```python
from build123d import *

# Parameters (mm, degrees)
BOSS_EXTRUDE1_DEPTH = 11.176
SKETCH2_R           = 2.032
CUT_EXTRUDE1_DEPTH  = 26.73462306
SKETCH4_W           = 2.54
SKETCH4_H           = 6.858
CUT_EXTRUDE2_DEPTH  = 0.508
SKETCH5_W           = 2.54
SKETCH5_H           = 6.858
CUT_EXTRUDE3_DEPTH  = 0.508


with BuildPart() as part:
    # Sketch1 → Boss-Extrude1 (new body)
    with BuildSketch(Plane.XY):
        with BuildLine():
            Line((8.39837008, 0), (21.09837008, 0))
            Line((21.09837008, 0), (21.09837008, 6.35))
            Line((21.09837008, 6.35), (21.60637008, 6.35))
            Line((21.60637008, 6.35), (21.60637008, -0.508))
            Line((21.60637008, -0.508), (7.874, -0.508))
            ThreePointArc((7.874, -0.508), (0, 7.89037008), (-7.874, -0.508))
            Line((-7.874, -0.508), (-21.60637008, -0.508))
            Line((-21.60637008, -0.508), (-21.60637008, 6.35))
            Line((-21.60637008, 6.35), (-21.09837008, 6.35))
            Line((-21.09837008, 6.35), (-21.09837008, 0))
            Line((-21.09837008, 0), (-8.39837008, 0))
            ThreePointArc((-8.39837008, 0), (0, 8.39837008), (8.39837008, 0))
        make_face()
    extrude(amount=BOSS_EXTRUDE1_DEPTH)

    # Sketch2 → Cut-Extrude1 (cut, through all)
    with BuildSketch(Plane(origin=(0, 0, 0), x_dir=(1, 0, 0), z_dir=(0, 1, 0))):
        with Locations(Location((15.00237008, -5.588, 0), (0, 0, 270))):
            Circle(SKETCH2_R)
        with Locations(Location((-15.00237008, -5.588, 0), (0, 0, 90))):
            Circle(SKETCH2_R)
    extrude(amount=-CUT_EXTRUDE1_DEPTH, mode=Mode.SUBTRACT)

    # Sketch4 → Cut-Extrude2 (cut)
    with BuildSketch(Plane(origin=(21.60637008, 0, 0), x_dir=(0, 0, -1), z_dir=(1, 0, 0))):
        with Locations((-5.207, 2.921)):
            Rectangle(SKETCH4_W, SKETCH4_H)
    extrude(amount=-CUT_EXTRUDE2_DEPTH, mode=Mode.SUBTRACT)

    # Sketch5 → Cut-Extrude3 (cut)
    with BuildSketch(Plane.ZY.offset(21.60637008)):
        with Locations((5.969, 2.921)):
            Rectangle(SKETCH5_W, SKETCH5_H)
    extrude(amount=-CUT_EXTRUDE3_DEPTH, mode=Mode.SUBTRACT)


solid = part.part
```
Geometry check sheet. Reference: the model listing, model coordinates, mm. A direction names the side the tool comes from. Give positions to 0.01 mm unless a question says otherwise; leave off trailing zeros. Loops run counter-clockwise (first coordinate to the right, second up) from the corner with the lowest first, then second, coordinate; pieces in that order, holes last. Notation, with made-up numbers: M 0.5,-28 L 10.5,-28 A17 cw 10.5,-7 Z; hole C 9.25,66 d3. An arc over 180 degrees is marked long. Write item = value, one per line. Start each with the question number.
1. Tool access check on faces 1 (the face through (-21.606, 3, 9)), 2 (the face through (-13, 0, 4)). Record the directions out of +Z, -Z, +X, -X, +Y, -Y that give a thin tool (end or side, any length) a straight path to the whole face; none if there is none.
2. Section check A-A, the plane z = 5.5. Enter the section's corners in (x, y).
3. Draft check along X on faces 3 (the face through (21.606, 3, 2)), 4 (the face through (-1, 8, 0)), 5 (the face through (-21.606, 3, 2)), 6 (the face through (21.098, 3, 2)). Enter one of: +X half, -X half, draft (parallel to the pull), parting line (faces both ways), or undercut.
4. Section check C-C, the plane z = 9.75. Enter the section's corners in (x, y), plus the area to 3 significant figures.
5. Thickness scan on probe 1 along X at (y, z) = (4.5, 3); probe 2 along X at (y, z) = (4.75, 2.5); probe 3 along Y at (x, z) = (18, 5.25). Record the ranges inside material, lowest first.
6. Section check B-B, the plane y = 5.25. Enter the section's corners in (x, z), plus the area to 3 significant figures.
7. Section check D-D, the plane y = 1.25. Enter the section's corners in (x, z), plus the area to 3 significant figures.
8. Go/stop test with flat-tipped pins: P1, Ø5.5, axis at x = -15.5, z = 7.5, coming from the +Y side; P2, Ø5, axis at y = 2, z = 4, coming from the +X side; P3, Ø1, axis at x = -1, z = 5.5, coming from the +Y side; P4, Ø1.5, axis at x = -3.5, z = 1.5, coming from the -Y side. Record where each tip stops, or that it passes through.
Values follow:
q1.face_1 = +Z, -Z, -X, +Y, -Y
q1.face_2 = +Z, -Z, +Y
q2.outline = M -21.1,-0.51 L -17.03,-0.51 L -17.03,0 L -21.1,0 Z; M -12.97,-0.51 L -7.87,-0.51 A7.89 cw long 7.87,-0.51 L 12.97,-0.51 L 12.97,0 L 8.4,0 A8.4 ccw -8.4,0 L -12.97,0 Z; M 17.03,-0.51 L 21.1,-0.51 L 21.1,0 L 17.03,0 Z
q3.face_3 = +X half
q3.face_4 = draft
q3.face_5 = -X half
q3.face_6 = undercut
q4.outline = M -21.61,-0.51 L -7.87,-0.51 A7.89 cw long 7.87,-0.51 L 21.61,-0.51 L 21.61,6.35 L 21.1,6.35 L 21.1,0 L 8.4,0 A8.4 ccw -8.4,0 L -21.1,0 L -21.1,6.35 L -21.61,6.35 Z
q4.area = 33.4 mm^2
q5.probe_1 = -21.61 to -21.1, -7.09 to -6.48, 6.48 to 7.09, 21.1 to 21.61
q5.probe_2 = -21.61 to -21.1, -6.93 to -6.3, 6.3 to 6.93, 21.1 to 21.61
q5.probe_3 = -0.51 to 0
q6.outline = M -21.61,0 L -21.1,0 L -21.1,4.7 L -21.61,4.7 Z; M -21.61,7.24 L -21.1,7.24 L -21.1,11.18 L -21.61,11.18 Z; M -6.56,0 L -5.89,0 L -5.89,11.18 L -6.56,11.18 Z; M 5.89,0 L 6.56,0 L 6.56,11.18 L 5.89,11.18 Z; M 21.1,0 L 21.61,0 L 21.61,3.94 L 21.1,3.94 Z; M 21.1,6.48 L 21.61,6.48 L 21.61,11.18 L 21.1,11.18 Z
q6.area = 23.6 mm^2
q7.outline = M -21.61,0 L -21.1,0 L -21.1,4.7 L -21.61,4.7 Z; M -21.61,7.24 L -21.1,7.24 L -21.1,11.18 L -21.61,11.18 Z; M -8.3,0 L -7.79,0 L -7.79,11.18 L -8.3,11.18 Z; M 7.79,0 L 8.3,0 L 8.3,11.18 L 7.79,11.18 Z; M 21.1,0 L 21.61,0 L 21.61,3.94 L 21.1,3.94 Z; M 21.1,6.48 L 21.61,6.48 L 21.61,11.18 L 21.1,11.18 Z
q7.area = 20.3 mm^2
q8.P1 = 0
q8.P2 = 21.61
q8.P3 = 8.38
q8.P4 = 6.65
